Here's how the part is built. I have some questions about the finished solid (model axes, mm). A direction names the side the tool comes from. Give positions to 0.01 mm unless a question says otherwise; leave off trailing zeros. Write each loop counter-clockwise with the first axis right and the second up, starting at its lowest first coordinate (ties: lowest second). Pieces come first, ordered by that corner, then holes. Notation, with made-up numbers: M -24,87.25 L 4,87.25 A35 ccw 4,124.25 Z; hole C -38.5,-10.5 d8. An arc over 180 degrees is marked long. Answer as CSV lines item,"result". Start each with the question number.
Q1. On a 3-axis mill with a long thin cutter (end or side, diameter ignored), from which of +Z, -Z, +X, -X, +Y, -Y can I reach the whole of each face in a straight line? I mean faces 1 (the flat face through (-25, 50, -38.1)), 2 (the flat face through (26, 101.6, 51)), 3 (the flat face through (12.7, 50, 51)). Say none if no direction works.
Q2. Suppose I cut it at A-A (y = 47). Write out the boundary of the cut face in (x, z), then the cut area to 3 significant figures.
Q3. For pin 1 (2 mm diameter, centred on x = -7, z = 23, fed in from +Y), with a flat end and sliding along its axis, tell me the tip position at first contact or that it passes through.
Q4. Suppose I cut it at D-D (z = 31.5). Write out the boundary of the cut face in (x, y).
Q5. If I drill on line 1 along X through (y, z) = (24.5, 43); line 2 along Z through (x, y) = (-26.5, 43.5); line 3 along Y through (x, z) = (17, 8.5), over which ranges is the centre line in solid material (lowest first)?
Q6. Suppose I cut it at C-C (z = -51). Write out the boundary of the cut face in (x, y).
Q7. Thinking about a two-plate mould opening in X: for faces 4 (the flat face through (-16, 24, 63.5)), 5 (the flat face through (-1, 0, 1)), 6 (the flat face through (38.1, -10, -1)), which applies, +X half, -X half, draft (parallel to the pull), parting line (faces both ways), or undercut?
Q8. Suppose I cut it at B-B (x = 32.5). Write out the boundary of the cut face in (y, z), then the cut area to 3 significant figures.
```python
from build123d import *

# Parameters (mm, degrees)
F0_W     = 76.2
F0_H     = 127
F1_DEPTH = 50.8
F2_W     = 25.4
F2_H     = 25.4
F3_DEPTH = 101.6
F4_DEPTH = 101.6


with BuildPart() as f1:
    # F0 (on Front) → F1 (new body)
    with BuildSketch(Plane.XZ):
        Rectangle(F0_W, F0_H)
    extrude(amount=F1_DEPTH)

    # F2 (on face) → F3 (join)
    with BuildSketch(Plane(origin=(0, 0, 0), x_dir=(-1, 0, 0), z_dir=(0, 1, 0))):
        with Locations((-25.4, 50.8)):
            Rectangle(F2_W, F2_H)
    extrude(amount=F3_DEPTH)

    # F2 (on face) → F4 (join)
    with BuildSketch(Plane(origin=(0, 0, 0), x_dir=(-1, 0, 0), z_dir=(0, 1, 0))):
        with Locations((25.4, 50.8)):
            Rectangle(F2_W, F2_H)
        with Locations((-25.4, 50.8)):
            Rectangle(F2_W, F2_H)
        with Locations((25.4, -50.8)):
            Rectangle(F2_W, F2_H)
        with Locations((-25.4, -50.8)):
            Rectangle(F2_W, F2_H)
    extrude(amount=F4_DEPTH)


solid = f1.part
```
Resolved:
1,face 1,"+X, -X, +Y"
1,face 2,"+Z, -Z, +X, -X, +Y"
1,face 3,"+Z, -Z, +Y"
2,outline,"M -38.1,-63.5 L -12.7,-63.5 L -12.7,-38.1 L -38.1,-38.1 Z; M -38.1,38.1 L -12.7,38.1 L -12.7,63.5 L -38.1,63.5 Z; M 12.7,-63.5 L 38.1,-63.5 L 38.1,-38.1 L 12.7,-38.1 Z; M 12.7,38.1 L 38.1,38.1 L 38.1,63.5 L 12.7,63.5 Z"
2,area,"2,580 mm^2"
3,pin 1,"y = 0"
4,outline,"M -38.1,-50.8 L 38.1,-50.8 L 38.1,0 L -38.1,0 Z"
5,line 1,"-38.1 to -12.7, 12.7 to 38.1"
5,line 2,"-63.5 to -38.1, 38.1 to 63.5"
5,line 3,"-50.8 to 0"
6,outline,"M -38.1,-50.8 L 38.1,-50.8 L 38.1,101.6 L 12.7,101.6 L 12.7,0 L -12.7,0 L -12.7,101.6 L -38.1,101.6 Z"
7,face 4,"draft"
7,face 5,"undercut"
7,face 6,"+X half"
8,outline,"M -50.8,-63.5 L 101.6,-63.5 L 101.6,-38.1 L 0,-38.1 L 0,38.1 L 101.6,38.1 L 101.6,63.5 L -50.8,63.5 Z"
8,area,"11,600 mm^2"
